For this review, use the dimensioned drawing (mm, ordinates from the lowest corner) and the shaded views. Coordinates: 2 decimals unless noted, no trailing zeros. Write each loop counter-clockwise with the first axis right and the second up, starting at its lowest first coordinate (ties: lowest second). Pieces come first, ordered by that corner, then holes. Notation, with made-up numbers: (-11.75, 76) - (31.25, 76) arc R15 ccw to (31.25, 101) - close; hole circle Ø1 at (77.5, -21). An arc over 180 degrees is marked (long way). Put each result on its own line as item: value.
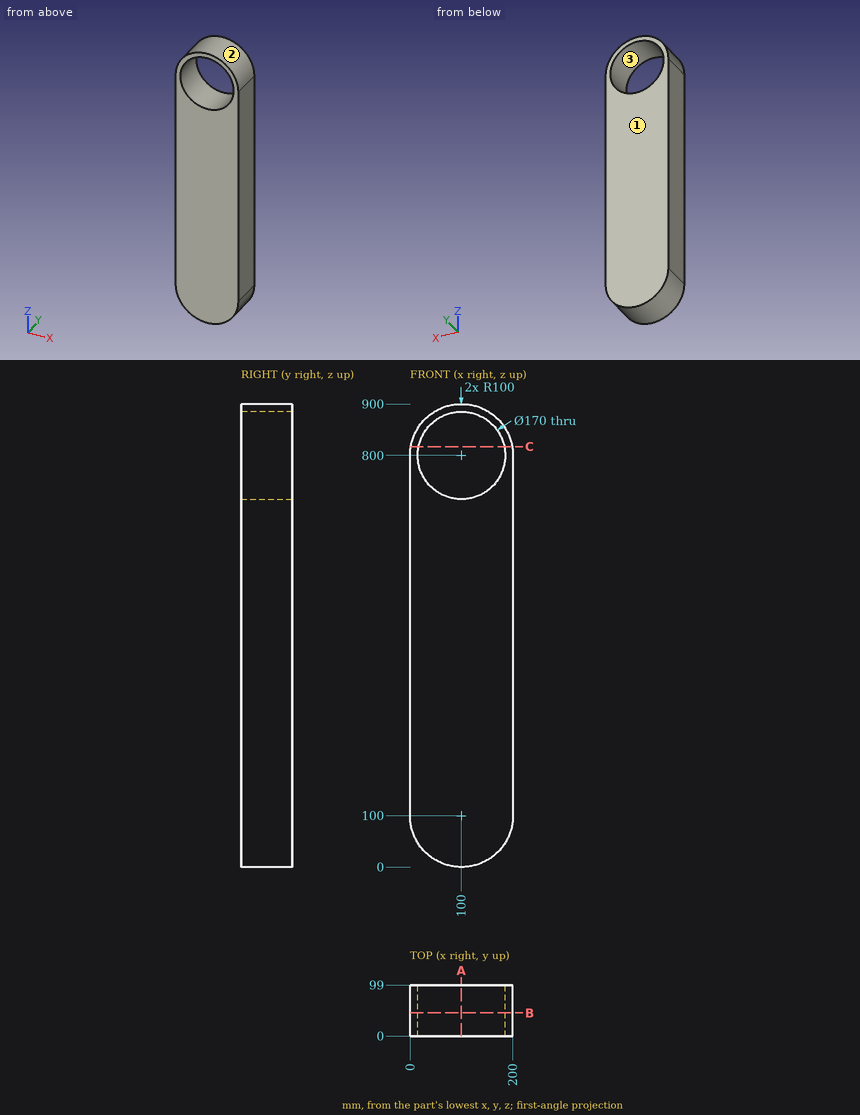
1. Consider section A-A on x = 100. State the section outline as (y, z) points.
Determined:
outline: (0, 0) - (99, 0) - (99, 715) - (0, 715) - close; (0, 885) - (99, 885) - (99, 900) - (0, 900) - close
2. For pin 1 Ø1.5 at (x, y) = (118.5, 26) entering from -Z; pin 2 Ø3 at (x, y) = (54.5, 80) entering from +Z, all flat-tipped, find the tip position at first contact; note any pin that passes through.
Determined:
pin 1: stops at z = 1.59
pin 2: stops at z = 889.8
3. To check wall thickness, follow probe 1 along X at (y, z) = (72.5, 800); probe 2 along Z at (x, y) = (148, 79.5); probe 3 along Z at (x, y) = (114.5, 66.5). State the ranges of each line that lie inside material, in increasing order.
Determined:
probe 1: x = 0 to 15, 185 to 200
probe 2: z = 12.27 to 729.85, 870.15 to 887.73
probe 3: z = 1.06 to 716.25, 883.75 to 898.94
4. Consider section C-C on z = 817. State the section outline as (x, y) points, plus the area to 3 significant figures.
Determined:
outline: (1.46, 0) - (16.72, 0) - (16.72, 99) - (1.46, 99) - close; (183.28, 0) - (198.54, 0) - (198.54, 99) - (183.28, 99) - close
area: 3,020 mm^2
5. The part is to be moulded in two halves that separate along Z. For the marked faces 1, 2 and 3, say which applies: +Z half, -Z half, draft (parallel to the pull), parting line (faces both ways), or undercut.
Determined:
face 1: draft
face 2: +Z half
face 3: undercut
6. Consider section B-B on y = 45. State the section outline as (x, z) points, plus the area to 3 significant figures.
Determined:
outline: (0, 100) arc R100 ccw to (200, 100) - (200, 800) arc R100 ccw to (0, 800) - close; hole circle Ø170 at (100, 800)
area: 149,000 mm^2
